Print and shaded views of the part. All mm, measured from the part's lowest x, y and z. Round coordinates to 2 decimals unless told otherwise and drop trailing zeros. Write each loop counter-clockwise with the first axis right and the second up, starting at its lowest first coordinate (ties: lowest second). Pieces come first, ordered by that corner, then holes. Notation, with made-up numbers: (89.25, 27) -> (97.25, 27) arc R7 cw to (97.25, 36) -> close; hole circle Ø11 at (81.5, -34). An arc over 180 degrees is marked (long way). Return JSON: item names as keys, results as strings. Group by question number.
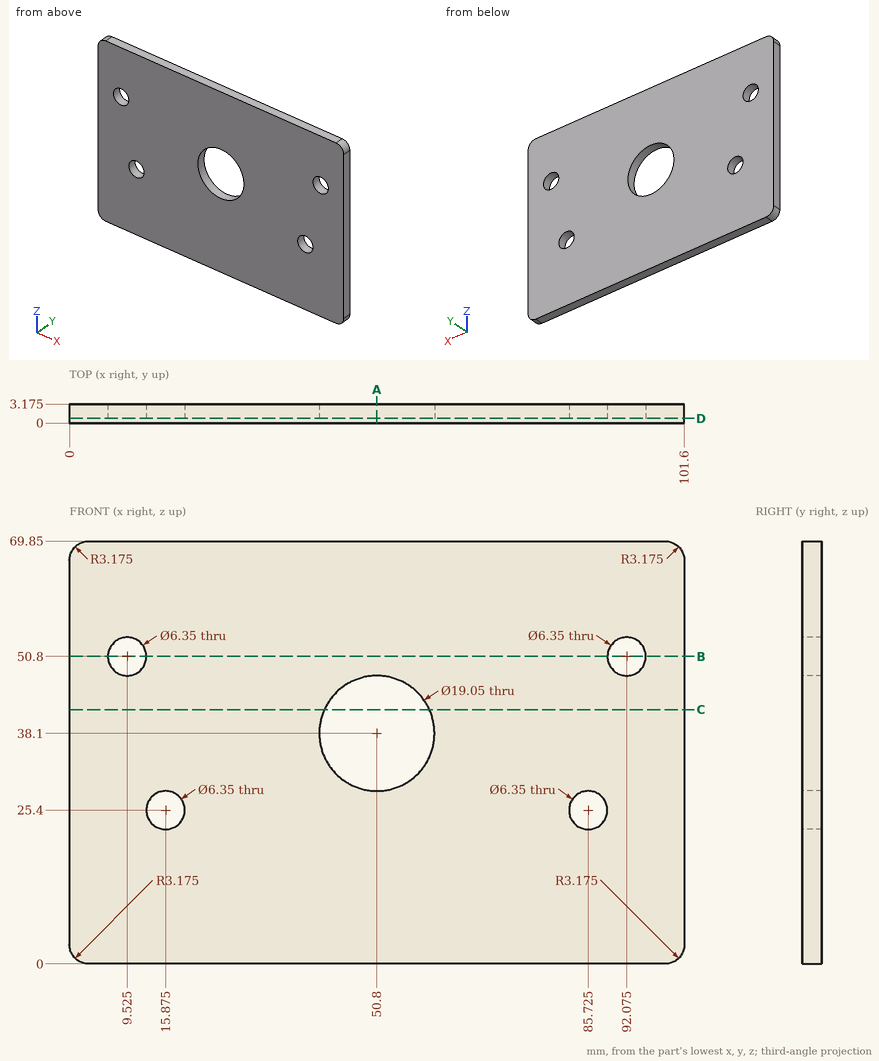
Item 1: Flat gauge pin, fed straight in: P1, Ø5.5, axis at x = 92.075, z = 50.8, coming from the +Y side. Where does the tip first touch, or does it go through?
Item 2: Cut at C-C (z = 42). Write the cut outline in (x, y) (3 decimals).
Item 3: Cut at D-D (y = 0.8). Write the cut outline in (x, z) (3 decimals), then the cut area to 3 significant figures.
Item 4: Cut at B-B (z = 50.8). Write the cut outline in (x, y) (3 decimals).
Item 5: Wall check: L1, parallel to X at y = 1.9, z = 50.8; L2, parallel to X at y = 1.5, z = 25; L3, parallel to Z at x = 51, y = 2.2. Give the ranges that are in metal, low to high.
Item 6: Cut at A-A (x = 50.8). Write the cut outline in (y, z) (3 decimals).
Checks:
{
 "1": {"P1": "passes through"},
 "2": {"outline": "(0, 0) -> (42.11, 0) -> (42.11, 3.175) -> (0, 3.175) -> close; (59.49, 0) -> (101.6, 0) -> (101.6, 3.175) -> (59.49, 3.175) -> close"},
 "3": {"outline": "(0, 3.175) arc R3.175 ccw to (3.175, 0) -> (98.425, 0) arc R3.175 ccw to (101.6, 3.175) -> (101.6, 66.675) arc R3.175 ccw to (98.425, 69.85) -> (3.175, 69.85) arc R3.175 ccw to (0, 66.675) -> close; hole circle Ø6.35 at (9.525, 50.8); hole circle Ø6.35 at (15.875, 25.4); hole circle Ø19.05 at (50.8, 38.1); hole circle Ø6.35 at (85.725, 25.4); hole circle Ø6.35 at (92.075, 50.8)", "area": "6,680 mm2"},
 "4": {"outline": "(0, 0) -> (6.35, 0) -> (6.35, 3.175) -> (0, 3.175) -> close; (12.7, 0) -> (88.9, 0) -> (88.9, 3.175) -> (12.7, 3.175) -> close; (95.25, 0) -> (101.6, 0) -> (101.6, 3.175) -> (95.25, 3.175) -> close"},
 "5": {"L1": "x = 0 to 6.35, 12.7 to 88.9, 95.25 to 101.6", "L2": "x = 0 to 12.73, 19.02 to 82.58, 88.87 to 101.6", "L3": "z = 0 to 28.58, 47.62 to 69.85"},
 "6": {"outline": "(0, 0) -> (3.175, 0) -> (3.175, 28.575) -> (0, 28.575) -> close; (0, 47.625) -> (3.175, 47.625) -> (3.175, 69.85) -> (0, 69.85) -> close"}
}
